Geometry: final body of the model. Coordinates: model frame, mm. Give positions to 0.01 mm unless a question says otherwise; leave off trailing zeros. Loops run counter-clockwise (first coordinate to the right, second up) from the corner with the lowest first, then second, coordinate; pieces in that order, holes last.
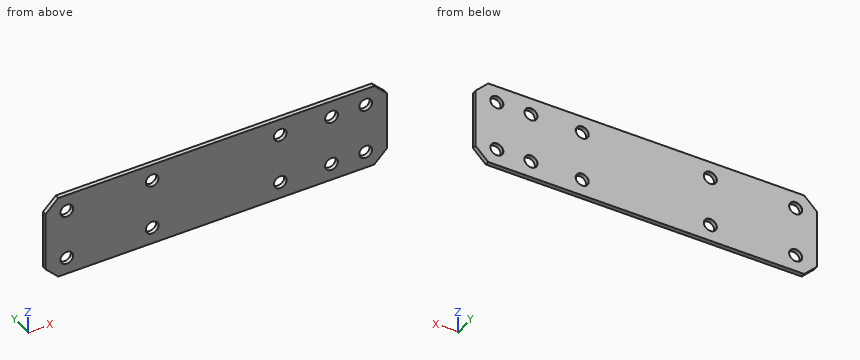
```python
from build123d import *

# Parameters (mm, degrees)
SKETCH_1_W            = 80
SKETCH_1_H            = 20
EXTRUDE_1_DEPTH       = 1
F_3_0MM_1_AT_2_COUNT  = 2
F_3_0MM_1_AT_2_PITCH  = 12
F_3_0MM_1_AT_3_COUNT  = 2
F_3_0MM_1_AT_3_PITCH  = 20
F_3_0MM_1_AT_4_COUNT  = 2
F_3_0MM_1_AT_4_PITCH  = 50
F_3_0MM_1_AT_5_COUNT  = 2
F_3_0MM_1_AT_5_PITCH  = 23.323807579
F_3_0MM_1_AT_6_COUNT  = 2
F_3_0MM_1_AT_6_PITCH  = 51.419840529
F_3_0MM_1_AT_7_COUNT  = 2
F_3_0MM_1_AT_7_PITCH  = 71.021123618
F_3_0MM_1_AT_8_COUNT  = 2
F_3_0MM_1_AT_8_PITCH  = 70
F_3_0MM_1_AT_9_COUNT  = 2
F_3_0MM_1_AT_9_PITCH  = 62
F_3_0MM_1_AT_10_COUNT = 2
F_3_0MM_1_AT_10_PITCH = 63.150613615
CHAMFER_1_SIZE        = 3


with BuildPart() as part:
    # 草图1 → 凸台-拉伸1 (new body)
    with BuildSketch(Plane(origin=(0, 0, 0), x_dir=(1, 0, 0), z_dir=(0, 1, 0))):
        with Locations((40, 10)):
            Rectangle(SKETCH_1_W, SKETCH_1_H)
    extrude(amount=EXTRUDE_1_DEPTH)

    # 草图3 → Ø3.0mm 暗销孔1 (revolve, cut)
    with BuildSketch(Plane(origin=(5, 1, -16), x_dir=(0, 0, 1), z_dir=(1, 0, 0))):
        Polygon((0, 0), (0, 1), (1.5, 1), (1.5, 0.025), (1.525, 0), align=None)
    f_3_0mm_1 = revolve(axis=Axis((5, 7.35, -16), (0, -1, 0)), mode=Mode.SUBTRACT)

    # Ø3.0mm 暗销孔1 at 2: Ø3.0mm 暗销孔1 ×2
    with Locations(*[(0, 0, i * F_3_0MM_1_AT_2_PITCH) for i in range(1, F_3_0MM_1_AT_2_COUNT)]):
        add(f_3_0mm_1, mode=Mode.SUBTRACT)

    # Ø3.0mm 暗销孔1 at 3: Ø3.0mm 暗销孔1 ×2
    with Locations(*[(i * F_3_0MM_1_AT_3_PITCH, 0, 0) for i in range(1, F_3_0MM_1_AT_3_COUNT)]):
        add(f_3_0mm_1, mode=Mode.SUBTRACT)

    # Ø3.0mm 暗销孔1 at 4: Ø3.0mm 暗销孔1 ×2
    with Locations(*[(i * F_3_0MM_1_AT_4_PITCH, 0, 0) for i in range(1, F_3_0MM_1_AT_4_COUNT)]):
        add(f_3_0mm_1, mode=Mode.SUBTRACT)

    # Ø3.0mm 暗销孔1 at 5: Ø3.0mm 暗销孔1 ×2
    with Locations(*[Vector(0.8574929257125442, 0, 0.5144957554275265) * (i * F_3_0MM_1_AT_5_PITCH) for i in range(1, F_3_0MM_1_AT_5_COUNT)]):
        add(f_3_0mm_1, mode=Mode.SUBTRACT)

    # Ø3.0mm 暗销孔1 at 6: Ø3.0mm 暗销孔1 ×2
    with Locations(*[Vector(0.9723873019805175, 0, 0.23337295247532422) * (i * F_3_0MM_1_AT_6_PITCH) for i in range(1, F_3_0MM_1_AT_6_COUNT)]):
        add(f_3_0mm_1, mode=Mode.SUBTRACT)

    # Ø3.0mm 暗销孔1 at 7: Ø3.0mm 暗销孔1 ×2
    with Locations(*[Vector(0.9856222548132667, 0, 0.1689638151108457) * (i * F_3_0MM_1_AT_7_PITCH) for i in range(1, F_3_0MM_1_AT_7_COUNT)]):
        add(f_3_0mm_1, mode=Mode.SUBTRACT)

    # Ø3.0mm 暗销孔1 at 8: Ø3.0mm 暗销孔1 ×2
    with Locations(*[(i * F_3_0MM_1_AT_8_PITCH, 0, 0) for i in range(1, F_3_0MM_1_AT_8_COUNT)]):
        add(f_3_0mm_1, mode=Mode.SUBTRACT)

    # Ø3.0mm 暗销孔1 at 9: Ø3.0mm 暗销孔1 ×2
    with Locations(*[(i * F_3_0MM_1_AT_9_PITCH, 0, 0) for i in range(1, F_3_0MM_1_AT_9_COUNT)]):
        add(f_3_0mm_1, mode=Mode.SUBTRACT)

    # Ø3.0mm 暗销孔1 at 10: Ø3.0mm 暗销孔1 ×2
    with Locations(*[Vector(0.9817798505902814, 0, 0.1900219065658609) * (i * F_3_0MM_1_AT_10_PITCH) for i in range(1, F_3_0MM_1_AT_10_COUNT)]):
        add(f_3_0mm_1, mode=Mode.SUBTRACT)

    # 倒角1
    chamfer_1_edges = [part.edges().sort_by_distance(p)[0] for p in [
        (0, 0.5, 0),
        (80, 0.5, 0),
        (80, 0.5, -20),
        (0, 0.5, -20),
    ]]
    chamfer(chamfer_1_edges, length=CHAMFER_1_SIZE)


solid = part.part
```
Q1. Section query B-B, the plane z = -4. State how many separate pieces and enclosed holes the cut face has, and give its area (3 significant figures).
Q2. Section query A-A, the plane x = 5. Return loops of the section in (y, z) (3 decimals).
Q3. Pin query (flat end, axial travel): pin 1 Ø5 at (x, z) = (67, -4) entering from +Y; pin 2 Ø2.5 at (x, z) = (67, -16) entering from -Y. Return the tip coordinate at first contact, or that it passes through.
Q4. Material intervals for probe 1 along Z at (x, y) = (5, 0.6); probe 2 along X at (y, z) = (0.5, -16); probe 3 along X at (y, z) = (0.65, -1.75), sorted ascending.
Resolved:
1. separate pieces: 6
1. enclosed holes: 0
1. area: 65.0 mm2
2. outline: (0, -20) - (1, -20) - (1, -17.525) - (0.975, -17.5) - (0, -17.5) - close; (0, -14.5) - (0.975, -14.5) - (1, -14.475) - (1, -5.525) - (0.975, -5.5) - (0, -5.5) - close; (0, -2.5) - (0.975, -2.5) - (1, -2.475) - (1, 0) - (0, 0) - close
3. pin 1: stops at y = 1
3. pin 2: passes through
4. probe 1: z = -20 to -17.5, -14.5 to -5.5, -2.5 to 0
4. probe 2: x = 0 to 3.5, 6.5 to 23.5, 26.5 to 53.5, 56.5 to 65.5, 68.5 to 73.5, 76.5 to 80
4. probe 3: x = 1.25 to 78.75
